```python
from build123d import *

# Parameters (mm, degrees)
F0_W      = 28.8499742746
F0_H      = 37.8827601671
F1_DEPTH  = 16
F2_DEPTH  = 296
F3_DEPTH  = 996
F4_W      = 199.8313069344
F4_H      = 801.1276721954
F5_DEPTH  = 5
F6_DEPTH  = 39.21
F7_DEPTH  = 2.24
F8_DEPTH  = 55.66
F9_DEPTH  = 1.59
F10_W     = 54.77245152
F10_H     = 895.9976721954
F11_DEPTH = 5
F12_DEPTH = 5.86
F13_DEPTH = 18.91
F14_W     = 83.0026693535
F14_H     = 34.9487662315
F14_H_2   = 55.274695158
F15_W     = 82.9961860609
F15_H     = 44.8832511902
F15_H_2   = 52.5203943253
F16_DEPTH = 5
F17_DEPTH = 300
F18_DEPTH = 300
F19_DEPTH = 324.79
F20_DEPTH = 324.79
F21_DEPTH = 250
F22_DEPTH = 250
F23_DEPTH = 100
F24_DEPTH = 100
F25_DEPTH = 50
F26_DEPTH = 50
F27_DEPTH = 134.02
F28_DEPTH = 100
F29_DEPTH = 100
F30_DEPTH = 100
F31_DEPTH = 50
F32_DEPTH = 54.95
F33_DEPTH = 50
F34_DEPTH = 109.29
F35_DEPTH = 14.88
F36_DEPTH = 230.15
F37_DEPTH = 230.15
F38_DEPTH = 22.52
F39_DEPTH = 77.2
F40_DEPTH = 77.2
F41_DEPTH = 11
F42_DEPTH = 200
F43_DEPTH = 200
F44_DEPTH = 200
F45_DEPTH = 70
F46_DEPTH = 70
F47_DEPTH = 70
F48_DEPTH = 70
F49_R     = 3


with BuildPart() as f1:
    # F0 (on Front) → F1 (new body)
    with BuildSketch(Plane.XZ):
        with Locations((14.4249871373, 18.9413800836)):
            Rectangle(F0_W, F0_H)
    extrude(amount=F1_DEPTH)

    # F2 (add): a face of the model
    f2_faces = [f1.faces().sort_by_distance(p)[0] for p in [
        (0, -8, 18.9413800836),
    ]]
    extrude(f2_faces, amount=-F2_DEPTH)

    # F3 (add): a face of the model
    f3_faces = [f1.faces().sort_by_distance(p)[0] for p in [
        (148, -8, 0),
    ]]
    extrude(f3_faces, amount=-F3_DEPTH)

    # F4 (on face) → F5 (cut)
    with BuildSketch(Plane.XZ.offset(16)):
        with Locations((148.3252942562, 506.2239170074)):
            Rectangle(F4_W, F4_H)
    extrude(amount=-F5_DEPTH, mode=Mode.SUBTRACT)

    # F6 (cut): a face of the model
    f6_faces = [f1.faces().sort_by_distance(p)[0] for p in [
        (148.3252942562, -13.5, 906.7877531052),
    ]]
    extrude(f6_faces, amount=-F6_DEPTH, mode=Mode.SUBTRACT)

    # F7 (add): a face of the model
    f7_faces = [f1.faces().sort_by_distance(p)[0] for p in [
        (248.2409477234, -13.5, 525.8289170074),
    ]]
    extrude(f7_faces, amount=F7_DEPTH)

    # F8 (cut): a face of the model
    f8_faces = [f1.faces().sort_by_distance(p)[0] for p in [
        (147.2052942562, -13.5, 105.6600809097),
    ]]
    extrude(f8_faces, amount=-F8_DEPTH, mode=Mode.SUBTRACT)

    # F9 (add): a face of the model
    f9_faces = [f1.faces().sort_by_distance(p)[0] for p in [
        (48.409640789, -13.5, 497.9989170074),
    ]]
    extrude(f9_faces, amount=F9_DEPTH)

    # F10 (on face) → F11 (join)
    with BuildSketch(Plane.XZ.offset(11)):
        with Locations((154.5285359025, 497.9989170074)):
            Rectangle(F10_W, F10_H)
    extrude(amount=F11_DEPTH)

    # F12 (cut): a face of the model
    f12_faces = [f1.faces().sort_by_distance(p)[0] for p in [
        (127.1423101425, -13.5, 497.9989170074),
    ]]
    extrude(f12_faces, amount=-F12_DEPTH, mode=Mode.SUBTRACT)

    # F13 (cut): a face of the model
    f13_faces = [f1.faces().sort_by_distance(p)[0] for p in [
        (181.9147616625, -13.5, 497.9989170074),
    ]]
    extrude(f13_faces, amount=-F13_DEPTH, mode=Mode.SUBTRACT)

    # F14 (on face) + F15 (on face) → F16 (join)
    with BuildSketch(Plane.XZ.offset(11)):
        with Locations((91.5009754658, 853.3093035221)):
            Rectangle(F14_W, F14_H)
        with Locations((91.5009754658, 511.6568356752)):
            Rectangle(F14_W, F14_H_2)
    with BuildSketch(Plane.XZ.offset(11)):
        with Locations((204.5028546929, 853.7013530731)):
            Rectangle(F15_W, F15_H)
        with Locations((204.5028546929, 576.5425562859)):
            Rectangle(F15_W, F15_H_2)
    extrude(amount=F16_DEPTH)

    # F17 (add): faces of the model
    f17_faces = [f1.faces().sort_by_distance(p)[0] for p in [
        (204.5028546929, -13.5, 550.2823591232),
        (91.5009754658, -13.5, 484.0194880962),
    ]]
    extrude(f17_faces, amount=F17_DEPTH)

    # F18 (cut): faces of the model
    f18_faces = [f1.faces().sort_by_distance(p)[0] for p in [
        (91.5009754658, -13.5, 539.2941832542),
        (204.5028546929, -13.5, 602.8027534485),
    ]]
    extrude(f18_faces, amount=-F18_DEPTH, mode=Mode.SUBTRACT)

    # F19 (add): a face of the model
    f19_faces = [f1.faces().sort_by_distance(p)[0] for p in [
        (91.5009754658, -13.5, 835.8349204063),
    ]]
    extrude(f19_faces, amount=F19_DEPTH)

    # F20 (cut): a face of the model
    f20_faces = [f1.faces().sort_by_distance(p)[0] for p in [
        (91.5009754658, -13.5, 870.7836866379),
    ]]
    extrude(f20_faces, amount=-F20_DEPTH, mode=Mode.SUBTRACT)

    # F21 (add): a face of the model
    f21_faces = [f1.faces().sort_by_distance(p)[0] for p in [
        (91.5009754658, -13.5, 239.2941832542),
    ]]
    extrude(f21_faces, amount=F21_DEPTH)

    # F22 (cut): a face of the model
    f22_faces = [f1.faces().sort_by_distance(p)[0] for p in [
        (91.5009754658, -13.5, 184.0194880962),
    ]]
    extrude(f22_faces, amount=-F22_DEPTH, mode=Mode.SUBTRACT)

    # F23 (add): a face of the model
    f23_faces = [f1.faces().sort_by_distance(p)[0] for p in [
        (91.5009754658, -13.5, 545.9936866379),
    ]]
    extrude(f23_faces, amount=F23_DEPTH)

    # F24 (cut): a face of the model
    f24_faces = [f1.faces().sort_by_distance(p)[0] for p in [
        (91.5009754658, -13.5, 511.0449204063),
    ]]
    extrude(f24_faces, amount=-F24_DEPTH, mode=Mode.SUBTRACT)

    # F25 (add): a face of the model
    f25_faces = [f1.faces().sort_by_distance(p)[0] for p in [
        (91.5009754658, -13.5, 645.9936866379),
    ]]
    extrude(f25_faces, amount=F25_DEPTH)

    # F26 (cut): a face of the model
    f26_faces = [f1.faces().sort_by_distance(p)[0] for p in [
        (91.5009754658, -13.5, 611.0449204063),
    ]]
    extrude(f26_faces, amount=-F26_DEPTH, mode=Mode.SUBTRACT)

    # F27 (add): a face of the model
    f27_faces = [f1.faces().sort_by_distance(p)[0] for p in [
        (91.5009754658, -13.5, 434.0194880962),
    ]]
    extrude(f27_faces, amount=F27_DEPTH)

    # F28 (cut): a face of the model
    f28_faces = [f1.faces().sort_by_distance(p)[0] for p in [
        (91.5009754658, -13.5, 299.9994880962),
    ]]
    extrude(f28_faces, amount=-F28_DEPTH, mode=Mode.SUBTRACT)

    # F29 (add): a face of the model
    f29_faces = [f1.faces().sort_by_distance(p)[0] for p in [
        (91.5009754658, -13.5, 661.0449204063),
    ]]
    extrude(f29_faces, amount=F29_DEPTH)

    # F30 (cut): a face of the model
    f30_faces = [f1.faces().sort_by_distance(p)[0] for p in [
        (91.5009754658, -13.5, 695.9936866379),
    ]]
    extrude(f30_faces, amount=-F30_DEPTH, mode=Mode.SUBTRACT)

    # F31 (add): a face of the model
    f31_faces = [f1.faces().sort_by_distance(p)[0] for p in [
        (91.5009754658, -13.5, 595.9936866379),
    ]]
    extrude(f31_faces, amount=F31_DEPTH)

    # F32 (cut): a face of the model
    f32_faces = [f1.faces().sort_by_distance(p)[0] for p in [
        (91.5009754658, -13.5, 561.0449204063),
    ]]
    extrude(f32_faces, amount=-F32_DEPTH, mode=Mode.SUBTRACT)

    # F33 (add): a face of the model
    f33_faces = [f1.faces().sort_by_distance(p)[0] for p in [
        (91.5009754658, -13.5, 399.9994880962),
    ]]
    extrude(f33_faces, amount=F33_DEPTH)

    # F34 (cut): a face of the model
    f34_faces = [f1.faces().sort_by_distance(p)[0] for p in [
        (91.5009754658, -13.5, 489.2941832542),
    ]]
    extrude(f34_faces, amount=-F34_DEPTH, mode=Mode.SUBTRACT)

    # F35 (cut): a face of the model
    f35_faces = [f1.faces().sort_by_distance(p)[0] for p in [
        (204.5028546929, -13.5, 831.259727478),
    ]]
    extrude(f35_faces, amount=-F35_DEPTH, mode=Mode.SUBTRACT)

    # F36 (add): a face of the model
    f36_faces = [f1.faces().sort_by_distance(p)[0] for p in [
        (204.5028546929, -13.5, 846.139727478),
    ]]
    extrude(f36_faces, amount=F36_DEPTH)

    # F37 (cut): a face of the model
    f37_faces = [f1.faces().sort_by_distance(p)[0] for p in [
        (204.5028546929, -13.5, 876.1429786682),
    ]]
    extrude(f37_faces, amount=-F37_DEPTH, mode=Mode.SUBTRACT)

    # F38 (cut): a face of the model
    f38_faces = [f1.faces().sort_by_distance(p)[0] for p in [
        (204.5028546929, -13.5, 250.2823591232),
    ]]
    extrude(f38_faces, amount=-F38_DEPTH, mode=Mode.SUBTRACT)

    # F39 (add): a face of the model
    f39_faces = [f1.faces().sort_by_distance(p)[0] for p in [
        (204.5028546929, -13.5, 302.8027534485),
    ]]
    extrude(f39_faces, amount=F39_DEPTH)

    # F40 (cut): a face of the model
    f40_faces = [f1.faces().sort_by_distance(p)[0] for p in [
        (204.5028546929, -13.5, 272.8023591232),
    ]]
    extrude(f40_faces, amount=-F40_DEPTH, mode=Mode.SUBTRACT)

    # F41 (cut): faces of the model
    f41_faces = [f1.faces().sort_by_distance(p)[0] for p in [
        (91.5009754658, -11, 795.9957198715),
        (204.5028546929, -11, 795.9953658867),
        (204.5028546929, -11, 497.9962404633),
        (91.5009754658, -11, 497.9995518303),
        (91.5009754658, -11, 199.999784503),
        (204.5028546929, -11, 200.0012200165),
    ]]
    extrude(f41_faces, amount=-F41_DEPTH, mode=Mode.SUBTRACT)

    # F42 (add): faces of the model
    f42_faces = [f1.faces().sort_by_distance(p)[0] for p in [
        (204.5028546929, -8, 615.989727478),
        (91.5009754658, -8, 615.9949204063),
    ]]
    extrude(f42_faces, amount=F42_DEPTH)

    # F43 (add): faces of the model
    f43_faces = [f1.faces().sort_by_distance(p)[0] for p in [
        (91.5009754658, -8, 945.9977531052),
        (204.5028546929, -8, 945.9977531052),
    ]]
    extrude(f43_faces, amount=F43_DEPTH)

    # F44 (cut): faces of the model
    f44_faces = [f1.faces().sort_by_distance(p)[0] for p in [
        (148, -8, 996),
        (91.5009754658, -8, 645.9936866379),
        (204.5028546929, -8, 645.9929786682),
    ]]
    extrude(f44_faces, amount=-F44_DEPTH, mode=Mode.SUBTRACT)

    # F45 (add): faces of the model
    f45_faces = [f1.faces().sort_by_distance(p)[0] for p in [
        (204.5028546929, -8, 350.0023591232),
        (91.5009754658, -8, 349.9994880962),
    ]]
    extrude(f45_faces, amount=F45_DEPTH)

    # F46 (cut): faces of the model
    f46_faces = [f1.faces().sort_by_distance(p)[0] for p in [
        (204.5028546929, -8, 380.0027534485),
        (91.5009754658, -8, 380.0041832542),
    ]]
    extrude(f46_faces, amount=-F46_DEPTH, mode=Mode.SUBTRACT)

    # F47 (add): faces of the model
    f47_faces = [f1.faces().sort_by_distance(p)[0] for p in [
        (204.5028546929, -8, 445.9929786682),
        (91.5009754658, -8, 445.9936866379),
    ]]
    extrude(f47_faces, amount=F47_DEPTH)

    # F48 (cut): faces of the model
    f48_faces = [f1.faces().sort_by_distance(p)[0] for p in [
        (204.5028546929, -8, 415.989727478),
        (91.5009754658, -8, 415.9949204063),
    ]]
    extrude(f48_faces, amount=-F48_DEPTH, mode=Mode.SUBTRACT)

    # F49
    f49_edges = [f1.edges().sort_by_distance(p)[0] for p in [
        (0, -16, 398),
        (148, -16, 0),
        (296, -16, 398),
        (148, -16, 796),
        (133.00231, -16, 164.999785),
        (91.500975, -16, 50.000081),
        (49.999641, -16, 164.999785),
        (91.500975, -16, 279.999488),
        (246.000948, -16, 165.00122),
        (204.502855, -16, 50.000081),
        (163.004762, -16, 165.00122),
        (204.502855, -16, 280.002359),
        (204.502855, -16, 310.002753),
        (163.004762, -16, 397.99624),
        (204.502855, -16, 485.989727),
        (246.000948, -16, 397.99624),
        (49.999641, -16, 397.999552),
        (91.500975, -16, 485.99492),
        (133.00231, -16, 397.999552),
        (91.500975, -16, 310.004183),
        (49.999641, -16, 630.99572),
        (91.500975, -16, 745.997753),
        (133.00231, -16, 630.99572),
        (91.500975, -16, 515.993687),
        (163.004762, -16, 630.995366),
        (204.502855, -16, 745.997753),
        (246.000948, -16, 630.995366),
        (204.502855, -16, 515.992979),
    ]]
    fillet(f49_edges, radius=F49_R)


solid = f1.part
```
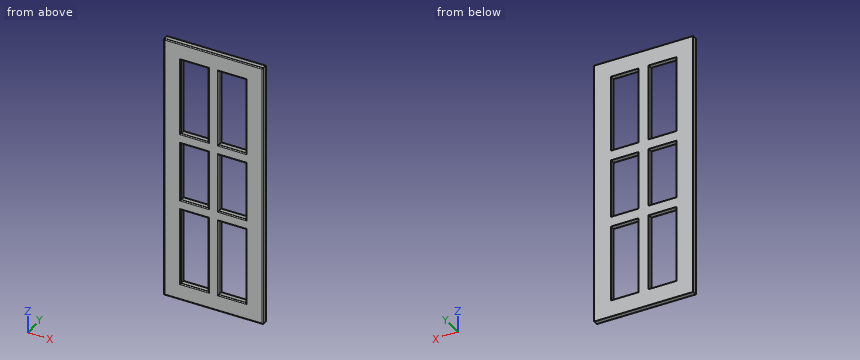
Work out the finished part from the listing and answer in its coordinate system (mm). Give positions to 0.01 mm unless a question says otherwise; leave off trailing zeros. Order: outer loops, then holes, each group sorted by start corner. A loop starts at its lowest first (then second) coordinate and runs counter-clockwise, first axis right, second up. Notation, with made-up numbers: M 3.5,24.5 L 56.5,24.5 A25 cw 56.5,52.5 Z; hole C 67.25,-34 d10. An arc over 180 degrees is marked long. Return JSON: item names as keys, results as strings.
1) Section C-C, the plane y = -3.5 is taken. Write down the section's boundary in (x, z).
Resolved:
{"outline": "M 0,0 L 296,0 L 296,796 L 0,796 Z; hole M 50,50 L 133,50 L 133,280 L 50,280 Z; hole M 50,310 L 133,310 L 133,485.99 L 50,485.99 Z; hole M 50,515.99 L 133,515.99 L 133,746 L 50,746 Z; hole M 163,50 L 246,50 L 246,280 L 163,280 Z; hole M 163,310 L 246,310 L 246,485.99 L 163,485.99 Z; hole M 163,515.99 L 246,515.99 L 246,746 L 163,746 Z"}
2) Straight lines are drawn through the part: line 1 along X through (y, z) = (-3.25, 467.5); line 2 along Z through (x, y) = (221, -6.75); line 3 along Z through (x, y) = (202, -15). For each, find the intervals that lie inside material, in ascending order. Write a range as [from, to].
Resolved:
{"line 1": "[0, 50], [133, 163], [246, 296]", "line 2": "[0, 50], [280, 310], [485.99, 515.99], [746, 796]", "line 3": "[0.76, 49.24], [280.77, 309.24], [486.75, 515.23], [746.76, 795.24]"}
3) Section A-A, the plane z = 343 is taken. Write down the section's boundary in (x, y), plus the area to 3 significant figures.
Resolved:
{"outline": "M 0,-13 A3 ccw 3,-16 L 47,-16 A3 ccw 50,-13 L 50,0 L 0,0 Z; M 133,-13 A3 ccw 136,-16 L 160,-16 A3 ccw 163,-13 L 163,0 L 133,0 Z; M 246,-13 A3 ccw 249,-16 L 293,-16 A3 ccw 296,-13 L 296,0 L 246,0 Z", "area": "2,070 mm^2"}
4) Section B-B, the plane x = 214.5 is taken. Write down the section's boundary in (y, z).
Resolved:
{"outline": "M -16,3 A3 ccw -13,0 L 0,0 L 0,50 L -13,50 A3 ccw -16,47 Z; M -16,283 A3 ccw -13,280 L 0,280 L 0,310 L -13,310 A3 ccw -16,307 Z; M -16,488.99 A3 ccw -13,485.99 L 0,485.99 L 0,515.99 L -13,515.99 A3 ccw -16,512.99 Z; M -16,749 A3 ccw -13,746 L 0,746 L 0,796 L -13,796 A3 ccw -16,793 Z"}
